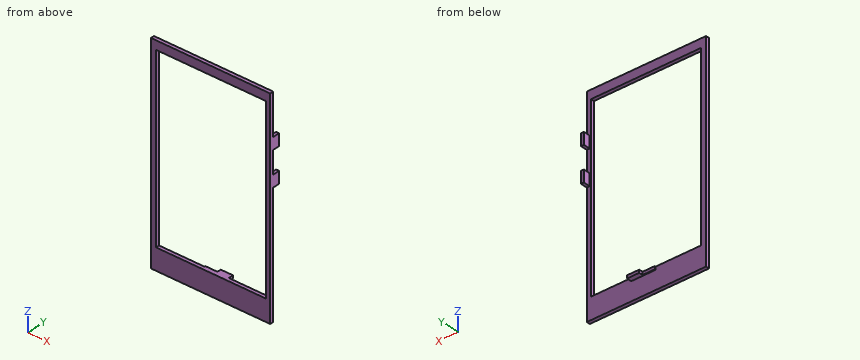
```python
from build123d import *

# Parameters (mm, degrees)
SKETCH1_W           = 56.06
SKETCH1_H           = 91.25
BOSS_EXTRUDE1_DEPTH = 1.8
BOSS_EXTRUDE2_DEPTH = 1.5
BOSS_EXTRUDE3_DEPTH = 1.5


with BuildPart() as part:
    # Sketch1 → Boss-Extrude1 (new body)
    # profile 1 of 2: a face of its own
    with BuildSketch(Plane(origin=(0, 0, 0), x_dir=(1, 0, 0), z_dir=(0, 1, 0))):
        Polygon((-30.193578772, 16.86607096), (30.606421228, 16.86607096), (30.606421228, -89.63392904), (-0.343578772, -89.63392904), (-30.193578772, -89.63392904), align=None)
        Polygon((-28.695861914, -88.133930777), (-28.695861914, 15.366069223), (29.104138086, 15.366069223), (29.104138086, -88.133930777), (-0.345861914, -88.133930777), align=None, mode=Mode.SUBTRACT)
    # profile 2 of 2: a face of its own
    with BuildSketch(Plane(origin=(0, 0, 0), x_dir=(1, 0, 0), z_dir=(0, 1, 0))):
        Polygon((-28.695861914, -88.133930777), (-0.345861914, -88.133930777), (29.104138086, -88.133930777), (29.104138086, 15.366069223), (-28.695861914, 15.366069223), align=None)
        with Locations((0.456421228, -39.58892904)):
            Rectangle(SKETCH1_W, SKETCH1_H, mode=Mode.SUBTRACT)
    extrude(amount=BOSS_EXTRUDE1_DEPTH)

    # Sketch4 → Boss-Extrude2 (add)
    with BuildSketch(Plane.XY.offset(-6.03607096)):
        Polygon((7.986421228, 1.8), (7.986421228, 4.3), (1.749686336, 4.3), (1.749686336, 2.3), (-4.513578772, 2.3), (-4.501292732, 1.8), (1.749686336, 1.8), align=None)
    extrude(amount=-BOSS_EXTRUDE2_DEPTH)

    # Sketch5 → Boss-Extrude3 (add)
    with BuildSketch(Plane(origin=(30.606421228, 0, 0), x_dir=(0, 0, -1), z_dir=(1, 0, 0))):
        Polygon((-68.657420773, 1.8), (-68.66392904, 5.3), (-62.66392904, 5.3), (-62.66392904, 1.8), align=None)
        Polygon((-51.24372118, 1.8), (-51.26392904, 5.3), (-45.26392904, 5.3), (-45.26392904, 1.8), align=None)
    extrude(amount=-BOSS_EXTRUDE3_DEPTH)


solid = part.part
```
Read the model definition and answer for the solid it produces. Units are mm, in the model's axes. Coordinates: 2 decimals unless noted, no trailing zeros. Write each loop counter-clockwise with the first axis right and the second up, starting at its lowest first coordinate (ties: lowest second). Pieces come first, ordered by that corner, then holes. Notation, with made-up numbers: (-35, 83.25) -> (5, 83.25) arc R28 ccw to (5, 101.25) -> close; hole circle Ø9 at (44.25, 5.5). An arc over 180 degrees is marked (long way). Return JSON: item names as keys, results as strings.
1. Find the intervals of material crossed by line 1 along Z through (x, y) = (18, 0.55); line 2 along X through (y, z) = (0.7, 14); line 3 along Y through (x, z) = (-13.5, -9), in increasing order. Write a range as from..to.
Found:
{"line 1": "-16.87..-6.04, 85.21..89.63", "line 2": "-30.19..-27.57, 28.49..30.61", "line 3": "0..1.8"}
2. A cutting plane is placed at D-D (y = 3.3). Determine the outline of the cut face in (x, z), and give its area (3 significant figures).
Found:
{"outline": "(1.75, -7.54) -> (7.99, -7.54) -> (7.99, -6.04) -> (1.75, -6.04) -> close; (29.11, 45.26) -> (30.61, 45.26) -> (30.61, 51.25) -> (29.11, 51.25) -> close; (29.11, 62.66) -> (30.61, 62.66) -> (30.61, 68.66) -> (29.11, 68.66) -> close", "area": "27.3 mm2"}
3. Each of these flat-tipped pins is pushed along its axis until it touches: P1, Ø0.8, axis at x = 2, y = 3, coming from the -Z side; P2, Ø1.6, axis at x = 30, y = 4, coming from the -Z side; P3, Ø1.8, axis at y = 3.5, z = 67, coming from the -X side. Where does it stop, or does it pass through?
Found:
{"P1": "z = -7.54", "P2": "z = 45.26", "P3": "x = 29.11"}
4. A cutting plane is placed at B-B (z = 5.5). Determine the outline of the cut face in (x, y).
Found:
{"outline": "(-30.19, 0) -> (-27.57, 0) -> (-27.57, 1.8) -> (-30.19, 1.8) -> close; (28.49, 0) -> (30.61, 0) -> (30.61, 1.8) -> (28.49, 1.8) -> close"}
5. A cutting plane is placed at C-C (z = 47). Determine the outline of the cut face in (x, y).
Found:
{"outline": "(-30.19, 0) -> (-27.57, 0) -> (-27.57, 1.8) -> (-30.19, 1.8) -> close; (28.49, 0) -> (30.61, 0) -> (30.61, 5.3) -> (29.11, 5.3) -> (29.11, 1.8) -> (28.49, 1.8) -> close"}
6. A cutting plane is placed at A-A (x = -9.5). Determine the outline of the cut face in (y, z).
Found:
{"outline": "(0, -16.87) -> (1.8, -16.87) -> (1.8, -6.04) -> (0, -6.04) -> close; (0, 85.21) -> (1.8, 85.21) -> (1.8, 89.63) -> (0, 89.63) -> close"}
